Geometry: final body of the model. Coordinates: model frame, mm. A direction names the side the tool comes from. Give positions to 0.01 mm unless a question says otherwise; leave off trailing zeros. Write each loop counter-clockwise with the first axis right and the second up, starting at its lowest first coordinate (ties: lowest second). Pieces come first, ordered by that corner, then holes.
Q1. Section D-D (x = 14). Return the cut outline in (y, z).
Q2. Section C-C (z = 39). Return the cut outline in (x, y), plus the area to 3 significant figures.
Q3. Reachability of faces 5 (the flat face through (25.4, 9, 15)), 6 (the flat face through (0, 19.05, 6)), 7 (the flat face through (12.7, -13, 6)), 8 (the flat face through (-6, 18.964, 26)), 9 (the flat face through (-6, 6.264, 26)) from +Z, -Z, +X, -X, +Y, -Y: full face, straight path, thin tool, end or side. Return the list, or none.
Q4. Pin query (flat end, axial travel): pin 1 Ø5 at (x, y) = (-7.5, 5) entering from -Z; pin 2 Ø4 at (x, z) = (20.5, 6.5) entering from -Y; pin 3 Ø1.5 at (x, z) = (14.5, 27.5) entering from +Y; pin 4 Ø12 at (x, z) = (6.5, 40) entering from -Y. Return the tip coordinate at first contact, or that it passes through.
Q5. Line query: line 1 (Z direction, x = 0, y = 14); line 2 (X direction, y = 14, z = 38); line 3 (Y direction, x = -17, z = 25). Output: solid intervals per line, ascending.
Q6. Mould query, pull axis Z, two halves, no side actions, for faces 1 (the flat face through (0, -6, 12.7)), 2 (the flat face through (-25.4, 8, 15)), 3 (the flat face through (0, 0, 0)), 4 (the cylindrical face through (-6.827, 12.703, 48.809)). Classes: +Z half, -Z half, draft (parallel to the pull), parting line (faces both ways), or undercut.
Q7. Section B-B (z = 9). Return the cut outline in (x, y).
Q8. Section A-A (x = -9). Return the cut outline in (y, z).
from build123d import *

# Parameters (mm, degrees)
F0_W     = 50.8
F0_H     = 38.1
F1_DEPTH = 12.7
F2_W     = 12.7
F2_H     = 12.7
F3_DEPTH = 12.7
F4_W     = 12.7
F4_H     = 50.8
F5_DEPTH = 50.8
F6_R     = 12.7
F7_DEPTH = 12.7
F8_R     = 25.4
F9_R     = 25.39999


# Not quite as in the source:
# - a fillet or chamfer is up to 0.001 mm smaller than in the source, because OpenCascade refuses the exact size


with BuildPart() as f1:
    # F0 (on Top) → F1 (new body)
    with BuildSketch(Plane.XY):
        Rectangle(F0_W, F0_H)
    extrude(amount=F1_DEPTH)

    # F2 (on face) → F3 (cut)
    with BuildSketch(Plane.XZ.offset(19.05)):
        with Locations((19.05, 6.35)):
            Rectangle(F2_W, F2_H)
    extrude(amount=-F3_DEPTH, mode=Mode.SUBTRACT)

    # F4 (on face) → F5 (join)
    with BuildSketch(Plane(origin=(-25.4, 0, 0), x_dir=(0, -1, 0), z_dir=(-1, 0, 0))):
        with Locations((-12.6142477781, 38.1)):
            Rectangle(F4_W, F4_H)
    extrude(amount=-F5_DEPTH)

    # F6 (on face) → F7 (cut)
    with BuildSketch(Plane(origin=(0, 18.9642477781, 0), x_dir=(-1, 0, 0), z_dir=(0, 1, 0))):
        with Locations((0, 38.1)):
            Circle(F6_R)
    extrude(amount=-F7_DEPTH, mode=Mode.SUBTRACT)

    # F8
    f8_edges = [f1.edges().sort_by_distance(p)[0] for p in [
        (-25.4, 12.614248, 63.5),
    ]]
    fillet(f8_edges, radius=F8_R)

    # F9 (radius 25.4 in the source; OpenCascade refuses exactly that, so slightly less here)
    f9_edges = [f1.edges().sort_by_distance(p)[0] for p in [
        (25.4, 12.614248, 63.5),
    ]]
    fillet(f9_edges, radius=F9_R)


solid = f1.part
Computed:
1. outline: (-6.35, 0) - (19.05, 0) - (19.05, 12.7) - (18.96, 12.7) - (18.96, 59.29) - (6.26, 59.29) - (6.26, 12.7) - (-6.35, 12.7) - close
2. outline: (-25.38, 6.26) - (-12.67, 6.26) - (-12.67, 18.96) - (-25.38, 18.96) - close; (12.67, 6.26) - (25.38, 6.26) - (25.38, 18.96) - (12.67, 18.96) - close
2. area: 323 mm2
3. face 5: +Z, -Z, +X, +Y, -Y
3. face 6: +Z, -Z, +X, -X, +Y
3. face 7: +Z, -Z, +X, -Y
3. face 8: +Z, +X, -X, +Y
3. face 9: +Z, +X, -X, -Y
4. pin 1: stops at z = 0
4. pin 2: stops at y = -6.35
4. pin 3: stops at y = 18.96
4. pin 4: stops at y = 6.26
5. line 1: z = 0 to 25.4, 50.8 to 63.5
5. line 2: x = -25.4 to -12.7, 12.7 to 25.4
5. line 3: y = 6.26 to 18.96
6. face 1: +Z half
6. face 2: draft
6. face 3: -Z half
6. face 4: undercut
7. outline: (-25.4, -19.05) - (12.7, -19.05) - (12.7, -6.35) - (25.4, -6.35) - (25.4, 19.05) - (-25.4, 19.05) - close
8. outline: (-19.05, 0) - (19.05, 0) - (19.05, 12.7) - (18.96, 12.7) - (18.96, 29.14) - (6.26, 29.14) - (6.26, 12.7) - (-19.05, 12.7) - close; (6.26, 47.06) - (18.96, 47.06) - (18.96, 61.85) - (6.26, 61.85) - close
